```python
from build123d import *


with BuildPart() as part:
    # 草图2 → 旋转2 (revolve)
    with BuildSketch(Plane(origin=(0, 0, 0), x_dir=(0, 0, -1), z_dir=(1, 0, 0)), mode=Mode.PRIVATE) as revolve_2_sk:
        with BuildLine():
            Line((1.6, 0), (4.5, 0))
            Line((4.5, 0), (4.5, 9))
            ThreePointArc((4.5, 9), (3.474873734, 11.474873734), (1, 12.5))
            Line((1, 12.5), (-2.5, 12.5))
            ThreePointArc((-2.5, 12.5), (-3.914213562, 11.914213562), (-4.5, 10.5))
            Line((-4.5, 10.5), (-4.4, 10.5))
            Line((-4.4, 10.5), (-4.4, 9.2))
            Line((-4.4, 9.2), (1.6, 9.2))
            Line((1.6, 9.2), (1.6, 0))
        make_face()
    revolve(revolve_2_sk.sketch.rotate(Axis((0, 0, -1.6), (0, 0, -1)), 180), axis=Axis((0, 0, -1.6), (0, 0, -1)))


solid = part.part
```
Could you check a few things on this model? Use its own coordinates, in mm. Round coordinates to 2 decimals unless told otherwise and drop trailing zeros. Order: outer loops, then holes, each group sorted by start corner. A loop starts at its lowest first (then second) coordinate and runs counter-clockwise, first axis right, second up. Notation, with made-up numbers: M 78,-4.5 L 119,-4.5 A24 ccw 119,24.5 Z; hole C 64,-3.75 d7. An arc over 180 degrees is marked long. One line per question, with ' | ' between items. Start each with the question number.
(1) Thinking about a two-plate mould opening in Y: for faces 1 (the face through (0, 0, -4.5)), 2 (the face through (-3.755, -11.923, 0.774)), 3 (the face through (0, 0, -1.6)), which applies, +Y half, -Y half, draft (parallel to the pull), parting line (faces both ways), or undercut?
(2) Please list where these lines run through material, in increasing order: line 1 along X through (y, z) = (0, -0.1); line 2 along Z through (x, y) = (-4.5, 7.25); line 3 along X through (y, z) = (4, 1.25).
(3) Suppose I cut it at D-D on z = -3. List the corners of the cut face in (x, y) for me.
(4) Suppose I cut it at A-A on x = 0. List the corners of the cut face in (y, z) for me.
(5) Suppose I cut it at C-C on z = -0.5. List the corners of the cut face in (x, y) for me, then the cut area to 3 significant figures.
(6) For P1, Ø2, axis at x = 2.5, z = 2, coming from the +Y side; P2, Ø1, axis at y = 2, z = 3, coming from the -X side; P3, Ø5.5, axis at x = 0, y = 0.5, coming from the +Z side, each with a flat end and sliding along its axis, tell me the tip position at first contact or that it passes through.
Geometry results:
1) face 1: draft | face 2: parting line | face 3: undercut
2) line 1: -12.5 to -9.2, 9.2 to 12.5 | line 2: -4.5 to -1.6 | line 3: -11.84 to -8.28, 8.28 to 11.84
3) outline: C 0,0 d23.74
4) outline: M -12.5,-1 A3.5 ccw -9,-4.5 L 9,-4.5 A3.5 ccw 12.5,-1 L 12.5,2.5 A2 ccw 10.5,4.5 L 10.5,4.4 L 9.2,4.4 L 9.2,-1.6 L -9.2,-1.6 L -9.2,4.4 L -10.5,4.4 L -10.5,4.5 A2 ccw -12.5,2.5 Z
5) outline: C 0,0 d25; hole C 0,0 d18.4 | area: 225 mm²
6) P1: y = 12.41 | P2: x = -12.39 | P3: z = -1.6
